Answer from the drawing. Dimensions are ordinates in mm from the lowest x, y and z of the part. Coordinates: 2 decimals unless noted, no trailing zeros. Write each loop counter-clockwise with the first axis right and the second up, starting at its lowest first coordinate (ties: lowest second). Pieces come first, ordered by that corner, then holes. Notation, with made-up numbers: (42.25, 34) -> (92.25, 34) arc R19 cw to (92.25, 55) -> close; hole circle Ø9 at (35, -5). An arc over 180 degrees is marked (long way). Use CSV: the item, a comma, the result in double quotes.
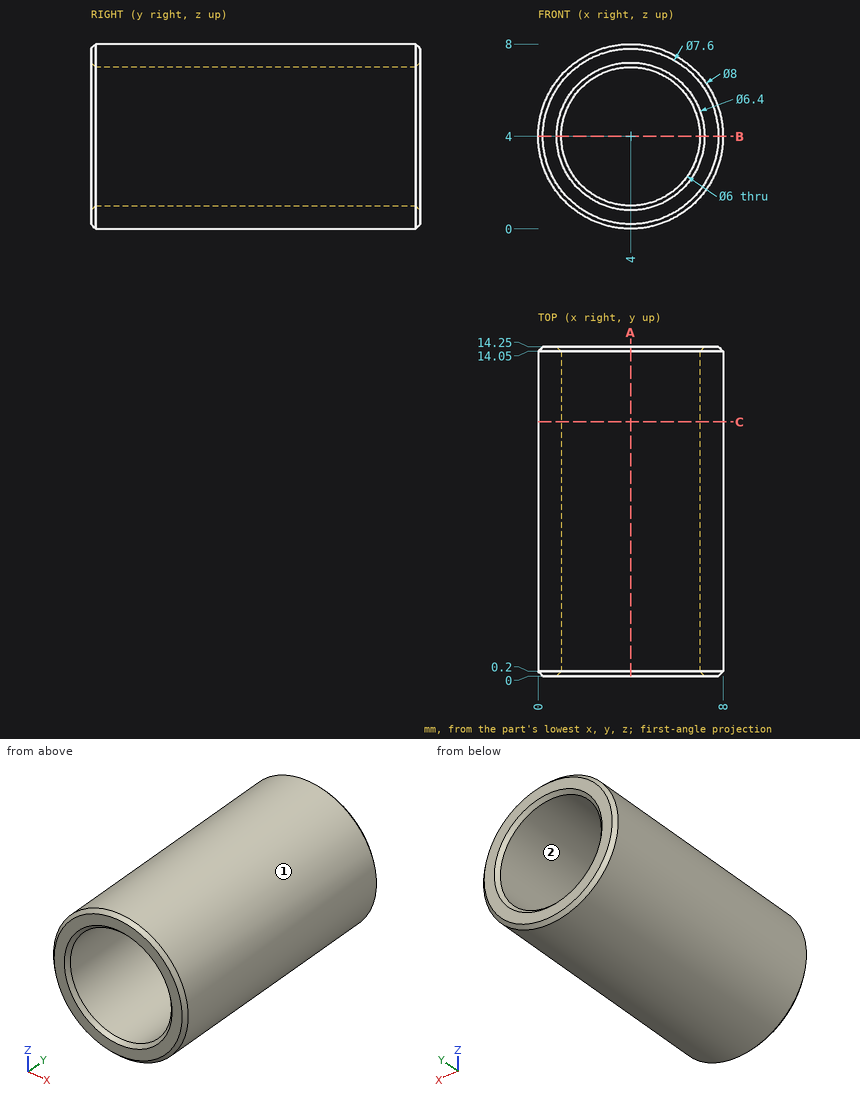
1. Find the intervals of material crossed by line 1 along X through (y, z) = (11.25, 4); line 2 along Z through (x, y) = (2.25, 11.5); line 3 along Z through (x, y) = (6, 11.5), in increasing order.
Solutions:
line 1,"x = 0 to 1, 7 to 8"
line 2,"z = 0.4 to 1.56, 6.44 to 7.6"
line 3,"z = 0.54 to 1.76, 6.24 to 7.46"
2. For a pull along Z with two mould halves and no side action, classify the marked faces 1 and 2 as pulls with the +Z half, pulls with the -Z half, needs draft (parallel to the pull), parting line crosses it, or undercut.
Solutions:
face 1,"parting line crosses it"
face 2,"undercut"
3. A cutting plane is placed at B-B (z = 4). Give the vertices of the cut face in (x, y), and give its area (3 significant figures).
Solutions:
outline,"(0, 0.2) -> (0.2, 0) -> (0.8, 0) -> (1, 0.2) -> (1, 14.05) -> (0.8, 14.25) -> (0.2, 14.25) -> (0, 14.05) -> close; (7, 0.2) -> (7.2, 0) -> (7.8, 0) -> (8, 0.2) -> (8, 14.05) -> (7.8, 14.25) -> (7.2, 14.25) -> (7, 14.05) -> close"
area,"28.3 mm^2"
4. A cutting plane is placed at A-A (x = 4). Give the vertices of the cut face in (y, z).
Solutions:
outline,"(0, 0.2) -> (0.2, 0) -> (14.05, 0) -> (14.25, 0.2) -> (14.25, 0.8) -> (14.05, 1) -> (0.2, 1) -> (0, 0.8) -> close; (0, 7.2) -> (0.2, 7) -> (14.05, 7) -> (14.25, 7.2) -> (14.25, 7.8) -> (14.05, 8) -> (0.2, 8) -> (0, 7.8) -> close"
5. Each of these flat-tipped pins is pushed along its axis until it touches: pin 1 Ø2 at (x, y) = (2.5, 4.5) entering from -Z; pin 2 Ø1.5 at (x, y) = (6, 8) entering from +Z; pin 3 Ø1 at (y, z) = (6.5, 5) entering from +X. Where does it stop, or does it pass through?
Solutions:
pin 1,"stops at z = 0.03"
pin 2,"stops at z = 7.8"
pin 3,"stops at x = 7.97"
6. A cutting plane is placed at C-C (y = 11). Give the vertices of the cut face in (x, z), and give its area (3 significant figures).
Solutions:
outline,"circle Ø8 at (4, 4); hole circle Ø6 at (4, 4)"
area,"22.0 mm^2"
